Part model, mm, in its own coordinate system. A direction names the side the tool comes from. Give positions to 0.01 mm unless a question says otherwise; leave off trailing zeros. Write each loop counter-clockwise with the first axis right and the second up, starting at its lowest first coordinate (ties: lowest second). Pieces come first, ordered by that corner, then holes.
```python
from build123d import *

# Parameters (mm, degrees)
EXTRUDE_1_DEPTH          = 40
CUT_EXTRUDE_1_REACH      = 43.207
CUT_EXTRUDE_1_END_RADIUS = 5.124355653
SKETCH_3_R               = 1.6
CUT_EXTRUDE_2_REACH      = 45.207
CUT_EXTRUDE_2_END_RADIUS = 5.124355653
CUT_EXTRUDE_START        = -2
SKETCH_4_R               = 3.75
CUT_EXTRUDE_3_REACH      = 43.207
EXTRUDE_2_REACH          = 42.93
CUT_EXTRUDE_4_REACH      = 43.207


with BuildPart() as part:
    # 草图1 → 凸台-拉伸1 (new body)
    with BuildSketch(Plane(origin=(0, 0, 0), x_dir=(1, 0, 0), z_dir=(0, 1, 0))):
        with BuildLine():
            Line((-4.437822174, -2.562177826), (-7, 1.875644347))
            Line((-7, 1.875644347), (7, 1.875644347))
            Line((7, 1.875644347), (4.437822174, -2.562177826))
            ThreePointArc((4.437822174, -2.562177826), (0, -5.124355653), (-4.437822174, -2.562177826))
        make_face()
    extrude(amount=EXTRUDE_1_DEPTH)

    # 切除-拉伸1: up to this cylinder (the profile starts inside it)
    cut_extrude_1_end = Plane(origin=(0, 20, 0), z_dir=(0, -1, 0)) * Cylinder(CUT_EXTRUDE_1_END_RADIUS, 129.662711306, mode=Mode.PRIVATE)
    # 草图3 → 切除-拉伸1 (cut, up to the surface)
    with BuildSketch(Plane(origin=(0, 0, -1.875644347), x_dir=(-1, 0, 0), z_dir=(0, 0, -1)), mode=Mode.PRIVATE) as cut_extrude_1_sk1:
        with Locations((0, 4)):
            Circle(SKETCH_3_R)
    cut_extrude_1_tool1 = extrude(cut_extrude_1_sk1.sketch, amount=-CUT_EXTRUDE_1_REACH, mode=Mode.PRIVATE) & cut_extrude_1_end
    add(cut_extrude_1_tool1.solids().sort_by_distance((0, 4, -1.875644))[0], mode=Mode.SUBTRACT)
    # 草图3 → 切除-拉伸1 (cut, up to the surface)
    with BuildSketch(Plane(origin=(0, 0, -1.875644347), x_dir=(-1, 0, 0), z_dir=(0, 0, -1)), mode=Mode.PRIVATE) as cut_extrude_1_sk2:
        with Locations((0, 36)):
            Circle(SKETCH_3_R)
    cut_extrude_1_tool2 = extrude(cut_extrude_1_sk2.sketch, amount=-CUT_EXTRUDE_1_REACH, mode=Mode.PRIVATE) & cut_extrude_1_end
    add(cut_extrude_1_tool2.solids().sort_by_distance((0, 36, -1.875644))[0], mode=Mode.SUBTRACT)

    # 切除-拉伸2: up to this cylinder (the profile starts inside it)
    cut_extrude_2_end = Plane(origin=(0, 20, 0), z_dir=(0, -1, 0)) * Cylinder(CUT_EXTRUDE_2_END_RADIUS, 133.662711306, mode=Mode.PRIVATE)
    # 草图4 → 切除-拉伸2 (cut, up to the surface)
    with BuildSketch(Plane(origin=(0, 0, -1.875644347), x_dir=(-1, 0, 0), z_dir=(0, 0, -1)).offset(CUT_EXTRUDE_START), mode=Mode.PRIVATE) as cut_extrude_2_sk1:
        with Locations((0, 4)):
            Circle(SKETCH_4_R)
    cut_extrude_2_tool1 = extrude(cut_extrude_2_sk1.sketch, amount=-CUT_EXTRUDE_2_REACH, mode=Mode.PRIVATE) & cut_extrude_2_end
    add(cut_extrude_2_tool1.solids().sort_by_distance((0, 4, 0.124356))[0], mode=Mode.SUBTRACT)
    # 草图4 → 切除-拉伸2 (cut, up to the surface)
    with BuildSketch(Plane(origin=(0, 0, -1.875644347), x_dir=(-1, 0, 0), z_dir=(0, 0, -1)).offset(CUT_EXTRUDE_START), mode=Mode.PRIVATE) as cut_extrude_2_sk2:
        with Locations((0, 36)):
            Circle(SKETCH_4_R)
    cut_extrude_2_tool2 = extrude(cut_extrude_2_sk2.sketch, amount=-CUT_EXTRUDE_2_REACH, mode=Mode.PRIVATE) & cut_extrude_2_end
    add(cut_extrude_2_tool2.solids().sort_by_distance((0, 36, 0.124356))[0], mode=Mode.SUBTRACT)

    # 草图6 → 切除-拉伸3 (cut, up to next)
    with BuildSketch(Plane(origin=(0, 0, -1.875644347), x_dir=(-1, 0, 0), z_dir=(0, 0, -1)), mode=Mode.PRIVATE) as cut_extrude_3_sk1:
        with BuildLine():
            Line((-7, 2), (-7, 0))
            Line((-7, 0), (-6.582575695, 0))
            ThreePointArc((-6.582575695, 0), (-6.894531565, 0.978451782), (-7, 2))
        make_face()
    cut_extrude_3_tool1 = extrude(cut_extrude_3_sk1.sketch, amount=-CUT_EXTRUDE_3_REACH, mode=Mode.PRIVATE) & part.part
    # 草图6 → 切除-拉伸3 (cut, up to next)
    with BuildSketch(Plane(origin=(0, 0, -1.875644347), x_dir=(-1, 0, 0), z_dir=(0, 0, -1)), mode=Mode.PRIVATE) as cut_extrude_3_sk2:
        with BuildLine():
            Line((-7, 40), (-6.582575695, 40))
            ThreePointArc((-6.582575695, 40), (-6.894531565, 39.021548218), (-7, 38))
            Line((-7, 38), (-7, 40))
        make_face()
    cut_extrude_3_tool2 = extrude(cut_extrude_3_sk2.sketch, amount=-CUT_EXTRUDE_3_REACH, mode=Mode.PRIVATE) & part.part
    add(cut_extrude_3_tool1.solids().sort_by_distance((6.875723, 0.49573, -1.875644))[0], mode=Mode.SUBTRACT)
    add(cut_extrude_3_tool2.solids().sort_by_distance((6.875723, 39.50427, -1.875644))[0], mode=Mode.SUBTRACT)

    # 凸台-拉伸2: up to this face of the body (flat: up to its plane)
    extrude_2_end = Plane(part.part.faces().sort_by_distance((-0.015198687, 40, 1.011851656))[0])
    # 草图7 → 凸台-拉伸2 (add, up to the picked face)
    with BuildSketch(Plane(origin=(0, 0, 0), x_dir=(1, 0, 0), z_dir=(0, 1, 0)), mode=Mode.PRIVATE) as extrude_2_sk1:
        Polygon((7, 1.875644347), (7, 4.875644347), (4, 1.875644347), align=None)
    extrude_2_tool1 = split(extrude(extrude_2_sk1.sketch, amount=EXTRUDE_2_REACH, mode=Mode.PRIVATE), bisect_by=extrude_2_end, keep=Keep.BOTH, mode=Mode.PRIVATE)
    add(extrude_2_tool1.solids().sort_by(Axis((6, 0, -2.875644), (0, 1, 0)))[0])

    # 切除-拉伸4: up to this plane
    cut_extrude_4_end = Plane(origin=(7, 44.242640687, -4.875644347), z_dir=(0.7071067811865476, 0, 0.7071067811865476))
    # 草图8 → 切除-拉伸4 (cut, up to the surface)
    with BuildSketch(Plane.XY.offset(-1.875644347), mode=Mode.PRIVATE) as cut_extrude_4_sk1:
        with BuildLine():
            Line((7, 38), (7, 40))
            Line((7, 40), (6.582575695, 40))
            ThreePointArc((6.582575695, 40), (6.894531565, 39.021548218), (7, 38))
        make_face()
    cut_extrude_4_tool1 = split(extrude(cut_extrude_4_sk1.sketch, amount=-CUT_EXTRUDE_4_REACH, mode=Mode.PRIVATE), bisect_by=cut_extrude_4_end, keep=Keep.BOTH, mode=Mode.PRIVATE)
    add(cut_extrude_4_tool1.solids().sort_by_distance((6.875723, 39.50427, -1.875644))[0], mode=Mode.SUBTRACT)
    # 草图8 → 切除-拉伸4 (cut, up to the surface)
    with BuildSketch(Plane.XY.offset(-1.875644347), mode=Mode.PRIVATE) as cut_extrude_4_sk2:
        with BuildLine():
            Line((6.582575695, 0), (7, 0))
            Line((7, 0), (7, 2))
            ThreePointArc((7, 2), (6.894531565, 0.978451782), (6.582575695, 0))
        make_face()
    cut_extrude_4_tool2 = split(extrude(cut_extrude_4_sk2.sketch, amount=-CUT_EXTRUDE_4_REACH, mode=Mode.PRIVATE), bisect_by=cut_extrude_4_end, keep=Keep.BOTH, mode=Mode.PRIVATE)
    add(cut_extrude_4_tool2.solids().sort_by_distance((6.875723, 0.49573, -1.875644))[0], mode=Mode.SUBTRACT)


solid = part.part
```
1) Saw through at A-A, the plane x = 0. Write the cut outline in (y, z), then the cut area to 3 significant figures.
Answers follow:
outline: (0, -1.88) - (2.4, -1.88) - (2.4, 0.12) - (0.25, 0.12) - (0.25, 5.12) - (0, 5.12) - close; (5.6, -1.88) - (34.4, -1.88) - (34.4, 0.12) - (32.25, 0.12) - (32.25, 5.12) - (7.75, 5.12) - (7.75, 0.12) - (5.6, 0.12) - close; (37.6, -1.88) - (40, -1.88) - (40, 5.12) - (39.75, 5.12) - (39.75, 0.12) - (37.6, 0.12) - close
area: 192 mm2
2) Saw through at D-D, the plane y = 13. Write the cut outline in (x, z).
Answers follow:
outline: (-7, -1.88) - (4, -1.88) - (7, -4.88) - (7, -1.88) - (4.44, 2.56) arc R5.12 ccw to (-4.44, 2.56) - close
3) Pin check, flat tips, straight feed: pin 1 Ø5 at (x, y) = (-3.5, 18) entering from +Z; pin 2 Ø1 at (y, z) = (13, 4) entering from -X; pin 3 Ø2 at (y, z) = (23.5, 3) entering from -X. Stop position of each tip, or through.
Answers follow:
pin 1: stops at z = 5.03
pin 2: stops at x = -3.74
pin 3: stops at x = -4.76
4) Saw through at B-B, the plane y = 36. Write the cut outline in (x, z).
Answers follow:
outline: (-7, -1.88) - (-1.6, -1.88) - (-1.6, 0.12) - (-3.75, 0.12) - (-3.75, 3.49) arc R5.12 ccw to (-4.44, 2.56) - close; (1.6, -1.88) - (4, -1.88) - (7, -4.88) - (7, -1.88) - (4.44, 2.56) arc R5.12 ccw to (3.75, 3.49) - (3.75, 0.12) - (1.6, 0.12) - close
5) Saw through at C-C, the plane z = -0.75. Write the cut outline in (x, y), then the cut area to 3 significant figures.
Answers follow:
outline: (-6.35, 0) - (6.35, 0) - (6.35, 40) - (-6.35, 40) - close; hole circle Ø3.2 at (0, 4); hole circle Ø3.2 at (0, 36)
area: 492 mm2
6) Wall check: L1, parallel to Y at x = 0, z = -1.3; L2, parallel to Y at x = 0, z = 1.6; L3, parallel to X at y = 6, z = 0.75. Give the ranges that are in metal, low to high.
Answers follow:
L1: y = 0 to 2.4, 5.6 to 34.4, 37.6 to 40
L2: y = 0 to 0.25, 7.75 to 32.25, 39.75 to 40
L3: x = -5.48 to -3.17, 3.17 to 5.48
7) 3-axis set-ups, long thin cutter, end or side, ignore diameter. For faces 1 (the face through (-2, 20, -1.876)), 2 (the face through (6.9, 1, -3.4)), 3 (the face through (0.81, 0.34, 2.04)): which of +Z, -Z, +X, -X, +Y, -Y reach the whole face in a straight line?
Answers follow:
face 1: -Z, -X, +Y, -Y
face 2: +Z, -Z, +X, -Y
face 3: +Z
8) Two-plate mould, pull along Y, no slides. Class faces 4 (the face through (5.521, 19.72, -3.397)), 5 (the face through (0, 0, 0)), 6 (the face through (-1.73, 32.673, 2.038)): +Y half, -Y half, draft (parallel to the pull), parting line (faces both ways), or undercut.
Answers follow:
face 4: draft
face 5: -Y half
face 6: undercut
